from build123d import *

# Parameters (mm, degrees)
F0_R     = 38.1
F1_DEPTH = 61.9125
F3_T     = -6.35


# Not quite as in the source:
# - a fillet or chamfer that OpenCascade refuses, or shapes differently, is made with other operations: its cross-section is extruded or revolved along the edge and cut away or added
# - a feature of the source that left no trace in its solid (it failed there, or was rolled back) is left out


with BuildPart() as f1:
    # F0 (on Front) → F1 (new body, symmetric)
    with BuildSketch(Plane.XZ):
        Circle(F0_R)
    extrude(amount=F1_DEPTH, both=True)

    # F3
    f3_openings = [f1.faces().sort_by_distance(p)[0] for p in [
        (0, -61.9125, 0),
    ]]
    offset(amount=F3_T, openings=f3_openings)

    # F4: fillet of radius 5.08 on 4 edges, made by hand

    # F4_s1 → F4_t2 (revolve)
    with BuildSketch(Plane.XY):
        with BuildLine():
            ThreePointArc((31.75, 50.4825), (30.2621024484, 54.0746024484), (26.67, 55.5625))
            Line((26.67, 55.5625), (31.75, 55.5625))
            Line((31.75, 55.5625), (31.75, 50.4825))
        make_face()
    revolve(axis=Axis((0, 55.5625, 0), (0, -1, 0)))

    # F4_s3 → F4_t4 (revolve, cut)
    with BuildSketch(Plane.XY):
        with BuildLine():
            ThreePointArc((38.1, -56.8325), (36.6121024484, -60.4246024484), (33.02, -61.9125))
            Line((33.02, -61.9125), (38.1, -61.9125))
            Line((38.1, -61.9125), (38.1, -56.8325))
        make_face()
    revolve(axis=Axis((0, -61.9125, 0), (0, -1, 0)), mode=Mode.SUBTRACT)

    # F4_s5 → F4_t6 (revolve, cut)
    with BuildSketch(Plane.XY):
        with BuildLine():
            ThreePointArc((33.02, -61.9125), (32.0780951188, -60.3484470592), (31.75, -58.5523958349))
            Line((31.75, -58.5523958349), (31.75, -61.9125))
            Line((31.75, -61.9125), (33.02, -61.9125))
        make_face()
    revolve(axis=Axis((0, -61.9125, 0), (0, -1, 0)), mode=Mode.SUBTRACT)


solid = f1.part
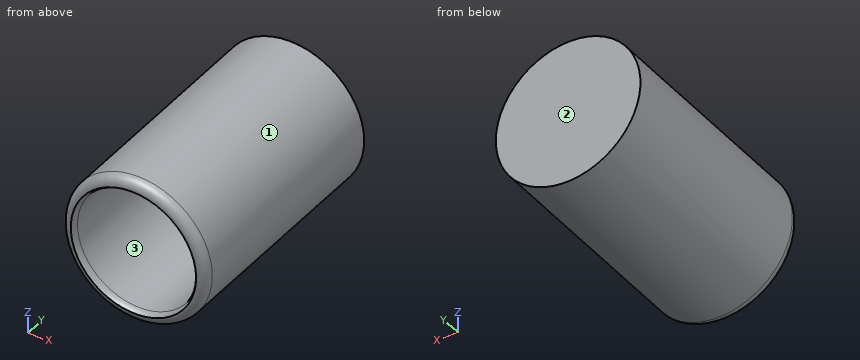
Build history of the part. All positions in model axes, mm. Face numbers are marked on the shaded views. Round coordinates to 2 decimals unless told otherwise and drop trailing zeros. Write each loop counter-clockwise with the first axis right and the second up, starting at its lowest first coordinate (ties: lowest second). Pieces come first, ordered by that corner, then holes. Notation, with made-up numbers: (-26.75, 14) -> (14.25, 14) arc R23 ccw to (14.25, 52) -> close; hole circle Ø1 at (-2.75, 68). An arc over 180 degrees is marked (long way). Write item = value, one per line.
(1) Band-saw the part on B-B (x = 0). Give the cut face in (y, z).
Answer:
outline = (-61.91, -33.02) arc R5.08 ccw to (-56.83, -38.1) -> (61.91, -38.1) -> (61.91, 38.1) -> (-56.83, 38.1) arc R5.08 ccw to (-61.91, 33.02) arc R5.08 ccw to (-58.55, 31.75) -> (50.48, 31.75) arc R5.08 cw to (55.56, 26.67) -> (55.56, -26.67) arc R5.08 cw to (50.48, -31.75) -> (-58.55, -31.75) arc R5.08 ccw to start
(2) Flat gauge pins, fed straight in: pin 1 (12 mm diameter, centred on x = -26, y = 31, fed in from +Z); pin 2 (12 mm diameter, centred on x = -13.5, y = -15, fed in from -Z); pin 3 (2 mm diameter, centred on x = -8.5, z = -20, fed in from -Y). Where does each tip first touch, or does it go through?
Answer:
pin_1 = 32.43
pin_2 = -37.35
pin_3 = 55.56
(3) Band-saw the part on C-C (y = 19). Give the cut face in (x, z), then the cut area to 3 significant figures.
Answer:
outline = circle Ø76.2 at (0, 0); hole circle Ø63.5 at (0, 0)
area = 1,390 mm2
(4) Band-saw the part on A-A (z = 0). Give the cut face in (x, y), then the cut area to 3 significant figures.
Answer:
outline = (-38.1, -56.83) arc R5.08 ccw to (-33.02, -61.91) arc R5.08 ccw to (-31.75, -58.55) -> (-31.75, 50.48) arc R5.08 cw to (-26.67, 55.56) -> (26.67, 55.56) arc R5.08 cw to (31.75, 50.48) -> (31.75, -58.55) arc R5.08 ccw to (33.02, -61.91) arc R5.08 ccw to (38.1, -56.83) -> (38.1, 61.91) -> (-38.1, 61.91) -> close
area = 1,970 mm2
(5) Probe L1, parallel to X at y = 30, z = -1; L2, parallel to Z at x = 0, y = 1; L3, parallel to Y at x = 19.5, z = -12.5. List the from-to ranges inside material, lowest first.
Answer:
L1 = -38.09 to -31.73, 31.73 to 38.09
L2 = -38.1 to -31.75, 31.75 to 38.1
L3 = 55.56 to 61.91
(6) Two-plate mould, pull along Z, no slides. Class the marked faces 1, 2 and 3: pulls with the +Z half, pulls with the -Z half, needs draft (parallel to the pull), parting line crosses it, or undercut.
Answer:
face_1 = parting line crosses it
face_2 = needs draft
face_3 = undercut
